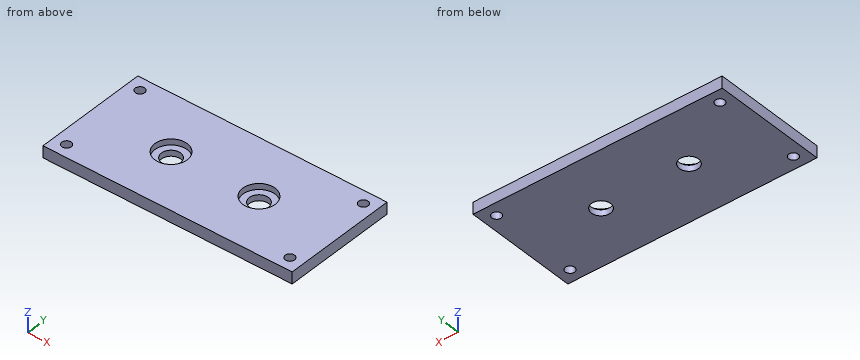
from build123d import *

# Parameters (mm, degrees)
SKETCH003_W     = 85
SKETCH003_H     = 39
PAD001_DEPTH    = 4
SKETCH007_R     = 1.6
SKETCH007_R_2   = 3.25
POCKET003_DEPTH = 5
SKETCH008_R     = 5.5
POCKET004_DEPTH = 2


with BuildPart() as part:
    # Sketch003 → Pad001 (new body)
    with BuildSketch(Plane.XY):
        Rectangle(SKETCH003_W, SKETCH003_H)
    extrude(amount=-PAD001_DEPTH)

    # Sketch007 → Pocket003 (cut)
    with BuildSketch(Plane.XY):
        with Locations((-38.1, 15.1)):
            Circle(SKETCH007_R)
        with Locations((-38.1, -15.1)):
            Circle(SKETCH007_R)
        with Locations((38.1, -15.1)):
            Circle(SKETCH007_R)
        with Locations((38.1, 15.1)):
            Circle(SKETCH007_R)
        with Locations((-15, 0)):
            Circle(SKETCH007_R_2)
        with Locations((15, 0)):
            Circle(SKETCH007_R_2)
    extrude(amount=-POCKET003_DEPTH, mode=Mode.SUBTRACT)

    # Sketch008 → Pocket004 (cut)
    with BuildSketch(Plane.XY):
        with Locations((-15, 0)):
            Circle(SKETCH008_R)
        with Locations((15, 0)):
            Circle(SKETCH008_R)
    extrude(amount=-POCKET004_DEPTH, mode=Mode.SUBTRACT)


solid = part.part
Could you check a few things on this model? Use its own coordinates, in mm. Round coordinates to 2 decimals unless told otherwise and drop trailing zeros. Loops run counter-clockwise (first coordinate to the right, second up) from the corner with the lowest first, then second, coordinate; pieces in that order, holes last. Notation, with made-up numbers: (-28.5, 72.5) -> (-22.5, 72.5) arc R17 ccw to (-22.5, 88.5) -> close; hole circle Ø5 at (-1, -16.75). An arc over 180 degrees is marked (long way). Use CSV: the item, a comma, the result in double quotes.
(1) If I drill on probe 1 along Y at (x, z) = (38.1, -1.2); probe 2 along Y at (x, z) = (-15, -2.6); probe 3 along X at (y, z) = (-1, -0.5), over which ranges is the centre line in solid material (lowest first)? Write a range as [from, to].
Return value:
probe 1,"y = [-19.5, -16.7], [-13.5, 13.5], [16.7, 19.5]"
probe 2,"y = [-19.5, -3.25], [3.25, 19.5]"
probe 3,"x = [-42.5, -20.41], [-9.59, 9.59], [20.41, 42.5]"
(2) Suppose I cut it at D-D on z = -2.95. Write out the boundary of the cut face in (x, y).
Return value:
outline,"(-42.5, -19.5) -> (42.5, -19.5) -> (42.5, 19.5) -> (-42.5, 19.5) -> close; hole circle Ø3.2 at (-38.1, -15.1); hole circle Ø3.2 at (-38.1, 15.1); hole circle Ø6.5 at (-15, 0); hole circle Ø6.5 at (15, 0); hole circle Ø3.2 at (38.1, -15.1); hole circle Ø3.2 at (38.1, 15.1)"
(3) Suppose I cut it at C-C on y = 15.1. Write out the boundary of the cut face in (x, z), plus the area to 3 significant figures.
Return value:
outline,"(-42.5, -4) -> (-39.7, -4) -> (-39.7, 0) -> (-42.5, 0) -> close; (-36.5, -4) -> (36.5, -4) -> (36.5, 0) -> (-36.5, 0) -> close; (39.7, -4) -> (42.5, -4) -> (42.5, 0) -> (39.7, 0) -> close"
area,"314 mm²"
(4) Suppose I cut it at A-A on x = 38.1. Write out the boundary of the cut face in (y, z), plus the area to 3 significant figures.
Return value:
outline,"(-19.5, -4) -> (-16.7, -4) -> (-16.7, 0) -> (-19.5, 0) -> close; (-13.5, -4) -> (13.5, -4) -> (13.5, 0) -> (-13.5, 0) -> close; (16.7, -4) -> (19.5, -4) -> (19.5, 0) -> (16.7, 0) -> close"
area,"130 mm²"
(5) Will this pin go through, and if not, where does the flat tip stop? pin 1 Ø1.9 at (x, y) = (-38.1, 15.1) entering from -Z.
Return value:
pin 1,"passes through"
(6) Suppose I cut it at B-B on x = 15. Write out the boundary of the cut face in (y, z), plus the area to 3 significant figures.
Return value:
outline,"(-19.5, -4) -> (-3.25, -4) -> (-3.25, -2) -> (-5.5, -2) -> (-5.5, 0) -> (-19.5, 0) -> close; (3.25, -4) -> (19.5, -4) -> (19.5, 0) -> (5.5, 0) -> (5.5, -2) -> (3.25, -2) -> close"
area,"121 mm²"
